from build123d import *

# Parameters (mm, degrees)
SKETCH1_R               = 49
SKETCH1_R_2             = 46
BOSS_EXTRUDE1_DEPTH     = 130
SKETCH2_R               = 1.5
CUT_EXTRUDE1_DEPTH      = 50
CUT_EXTRUDE1_DEPTH_BACK = 50
SKETCH3_R               = 9.5
CUT_EXTRUDE2_DEPTH      = 50.000000109
CUT_EXTRUDE2_DEPTH_BACK = 50.000000109
SKETCH4_R               = 1.5
CUT_EXTRUDE3_DEPTH      = 50.000000109
CUT_EXTRUDE3_DEPTH_BACK = 50.000000109
CUT_EXTRUDE4_DEPTH      = 70
CUT_EXTRUDE4_DEPTH_BACK = 70


with BuildPart() as part:
    # Sketch1 → Boss-Extrude1 (new body)
    with BuildSketch(Plane(origin=(0, 0, 0), x_dir=(1, 0, 0), z_dir=(0, 1, 0))):
        Circle(SKETCH1_R)
        Circle(SKETCH1_R_2, mode=Mode.SUBTRACT)
    extrude(amount=BOSS_EXTRUDE1_DEPTH)

    # Sketch2 → Cut-Extrude1 (cut, two sides)
    with BuildSketch(Plane.XY) as cut_extrude1_sk:
        with Locations((0, 11.4)):
            Circle(SKETCH2_R)
    extrude(amount=CUT_EXTRUDE1_DEPTH, mode=Mode.SUBTRACT)
    extrude(cut_extrude1_sk.sketch, amount=-CUT_EXTRUDE1_DEPTH_BACK, mode=Mode.SUBTRACT)

    # Sketch3 → Cut-Extrude2 (cut, two sides)
    with BuildSketch(Plane.XY) as cut_extrude2_sk:
        with Locations((0, 100)):
            Circle(SKETCH3_R)
    extrude(amount=CUT_EXTRUDE2_DEPTH, mode=Mode.SUBTRACT)
    extrude(cut_extrude2_sk.sketch, amount=-CUT_EXTRUDE2_DEPTH_BACK, mode=Mode.SUBTRACT)

    # Sketch4 → Cut-Extrude3 (cut, two sides)
    with BuildSketch(Plane.XY) as cut_extrude3_sk:
        with Locations((0, 83.5)):
            Circle(SKETCH4_R)
        with Locations((0, 116.5)):
            Circle(SKETCH4_R)
    extrude(amount=CUT_EXTRUDE3_DEPTH, mode=Mode.SUBTRACT)
    extrude(cut_extrude3_sk.sketch, amount=-CUT_EXTRUDE3_DEPTH_BACK, mode=Mode.SUBTRACT)

    # Sketch5 → Cut-Extrude4 (cut, two sides)
    with BuildSketch(Plane(origin=(0, 0, 0), x_dir=(0, 0, -1), z_dir=(1, 0, 0))) as cut_extrude4_sk:
        Polygon((0, 70), (2, 70), (2, 130), (-2, 130), (-2, 70), align=None)
    extrude(amount=CUT_EXTRUDE4_DEPTH, mode=Mode.SUBTRACT)
    extrude(cut_extrude4_sk.sketch, amount=-CUT_EXTRUDE4_DEPTH_BACK, mode=Mode.SUBTRACT)


solid = part.part
For this review, take the finished solid that the model builds, in its own axes (mm). A direction names the side the tool comes from. Give positions to 0.01 mm unless a question says otherwise; leave off trailing zeros. Order: outer loops, then holes, each group sorted by start corner. A loop starts at its lowest first (then second) coordinate and runs counter-clockwise, first axis right, second up. Notation, with made-up numbers: M 26.25,-39.75 L 72.25,-39.75 A36 cw 72.25,-2.75 Z; hole C -34,-30 d2. An arc over 180 degrees is marked long. Answer in a Markdown table with one row per item. Add a question column.
(1) For faces 1 (the face through (0, 85, 47)), 2 (the face through (-47, 100, -2)), list the 3-axis set-ups (+Z, -Z, +X, -X, +Y, -Y) from which the entire face can be reached by the end or side of a thin tool; tool diameter is ignored.
(2) Consider section D-D on y = 64.5. State the section outline as (x, z) points.
(3) Consider section A-A on x = 34. State the section outline as (y, z) points.
(4) Consider section C-C on z = 16. State the section outline as (x, y) points.
(5) Wall thickness on probe 1 along Y at (x, z) = (0, 47.2); probe 2 along Z at (x, y) = (1, 46); probe 3 along Z at (x, y) = (30, 75): over which ranges is each line inside the solid? List them lowest first. Write a range as [from, to].
(6) Consider section B-B on y = 94. State the section outline as (x, z) points, and give its area (3 significant figures).
(7) For pin 1 (3.5 mm diameter, centred on x = 47.5, z = 0, fed in from +Y); pin 2 (10 mm diameter, centred on x = -26, y = 92.5, fed in from -Z); pin 3 (12 mm diameter, centred on x = 22.5, y = 23, fed in from -Z), all flat-tipped, find the tip position at first contact; note any pin that passes through.
(8) Mouldability with a two-part tool opening along Y and no side actions: class faces 3 (the face through (-47, 100, 2)), 4 (the face through (-47, 70, 0)), 5 (the face through (-7.54, 94.22, 46.98)) as +Y half, -Y half, draft (parallel to the pull), parting line (faces both ways), or undercut.
Evaluation:
| question | item | result |
|---|---|---|
| 1 | face 1 | +Z, -Z |
| 1 | face 2 | +X, -X, +Y |
| 2 | outline | C 0,0 d98; hole C 0,0 d92 |
| 3 | outline | M 0,-35.28 L 130,-35.28 L 130,-30.98 L 0,-30.98 Z; M 0,30.98 L 130,30.98 L 130,35.28 L 0,35.28 Z |
| 4 | outline | M -46.31,0 L -43.13,0 L -43.13,130 L -46.31,130 Z; M 43.13,0 L 46.31,0 L 46.31,130 L 43.13,130 Z |
| 5 | probe 1 | y = [0, 9.9], [12.9, 82], [85, 90.5], [109.5, 115], [118, 130] |
| 5 | probe 2 | z = [-48.99, -45.99], [45.99, 48.99] |
| 5 | probe 3 | z = [-38.74, -34.87], [34.87, 38.74] |
| 6 | outline | M -48.96,-2 A49 ccw -7.37,-48.44 L -7.37,-45.41 A46 cw -45.96,-2 Z; M -48.96,2 L -45.96,2 A46 cw -7.37,45.41 L -7.37,48.44 A49 ccw Z; M 7.37,-48.44 A49 ccw 48.96,-2 L 45.96,-2 A46 cw 7.37,-45.41 Z; M 7.37,45.41 A46 cw 45.96,2 L 48.96,2 A49 ccw 7.37,48.44 Z |
| 6 | area | 783 mm^2 |
| 7 | pin 1 | stops at y = 70 |
| 7 | pin 2 | stops at z = -44.27 |
| 7 | pin 3 | stops at z = -46.14 |
| 8 | face 3 | draft |
| 8 | face 4 | +Y half |
| 8 | face 5 | undercut |
